Build history of the part. All positions in model axes, mm. A direction names the side the tool comes from. Give positions to 0.01 mm unless a question says otherwise; leave off trailing zeros. Use a Markdown table: item, result. Add a question column.
(1) Mould opens along Y. For faces 1 (the face through (30, 12, 40)), 2 (the face through (-0.901, -75.004, 24.79)), 3 (the face through (0.901, 75.004, 24.79)), 4 (the face through (-42.222, 32.375, 25.243)) say: +Y half, -Y half, draft (parallel to the pull), parting line (faces both ways), or undercut.
(2) Slice it at C-C (x = 69). Count the separate pieces of the cut face and the enclosed holes in it, then the cut area to 3 significant figures.
(3) Which spindle directions (+Z, -Z, +X, -X, +Y, -Y) get a long thin tool onto all of the face, cutting with end or side? Do faces 5 (the face through (-85.82, 0.79, 16.79)), 6 (the face through (92.5, -1, 7)), 7 (the face through (85.572, 0.791, 16.856)), 8 (the face through (-66.18, 86.51, 25.65)). Say none if no direction does.
(4) Wall check: line 1 (X direction, y = -86, z = 27); line 2 (Y direction, x = -64.5, z = 22); line 3 (X direction, y = -72, z = 4.5). Give the ranges that are in metal, low to high.
(5) Flat gauge pins, fed straight in: pin 1 (1.5 mm diameter, centred on x = 31.5, z = 6, fed in from -Y); pin 2 (10.5 mm diameter, centred on x = 75, y = 75, fed in from +Z); pin 3 (7.5 mm diameter, centred on y = 25, z = 11, fed in from -X); pin 4 (14.5 mm diameter, centred on x = 77, y = 74.5, fed in from +Z). Where does each tip first touch, or does it go through?
from build123d import *

# Parameters (mm, degrees)
SKETCH1_R                       = 25
BOSS_EXTRUDE1_DEPTH             = 30
SKETCH2_W                       = 185
SKETCH2_H                       = 185
BOSS_EXTRUDE2_DEPTH             = 15
DRAFT1_ANGLE                    = 15
DRAFT2_ANGLE                    = 15
DRAFT3_ANGLE                    = 15
DRAFT4_ANGLE                    = 15
SKETCH3_R                       = 42.5
BOSS_EXTRUDE3_DEPTH             = 40
CBORE_FOR_M16_SBHCS1_AT_2_COUNT = 2
CBORE_FOR_M16_SBHCS1_AT_2_PITCH = 150
CBORE_FOR_M16_SBHCS1_AT_3_COUNT = 2
CBORE_FOR_M16_SBHCS1_AT_3_PITCH = 150
CBORE_FOR_M16_SBHCS1_AT_4_COUNT = 2
CBORE_FOR_M16_SBHCS1_AT_4_PITCH = 212.132034356
SKETCH6_R                       = 30
CUT_EXTRUDE1_DEPTH              = 147.969384567
SKETCH7_R                       = 77.5
CUT_EXTRUDE2_DEPTH              = 5
FILLET1_R                       = 3
CHAMFER1_SIZE                   = 2


with BuildPart() as part:
    # Sketch1 → Boss-Extrude1 (new body)
    with BuildSketch(Plane.XY):
        with BuildLine():
            ThreePointArc((-60, 95), (-52.639320225, 86.180339887), (-50, 75))
            ThreePointArc((-50, 75), (-67.09430585, 51.282917549), (-95, 60))
            ThreePointArc((-95, 60), (-75, 0), (-95, -60))
            ThreePointArc((-95, -60), (-67.09430585, -51.282917549), (-50, -75))
            ThreePointArc((-50, -75), (-52.639320225, -86.180339887), (-60, -95))
            ThreePointArc((-60, -95), (0, -75), (60, -95))
            ThreePointArc((60, -95), (57.32233047, -57.32233047), (95, -60))
            ThreePointArc((95, -60), (75, 0), (95, 60))
            ThreePointArc((95, 60), (57.32233047, 57.32233047), (60, 95))
            ThreePointArc((60, 95), (0, 75), (-60, 95))
        make_face()
        with Locations((-75, 75)):
            Circle(SKETCH1_R)
        with Locations((75, 75)):
            Circle(SKETCH1_R)
        with Locations((75, -75)):
            Circle(SKETCH1_R)
        with Locations((-75, -75)):
            Circle(SKETCH1_R)
    extrude(amount=BOSS_EXTRUDE1_DEPTH)

    # Sketch2 → Boss-Extrude2 (add)
    with BuildSketch(Plane.XY):
        Rectangle(SKETCH2_W, SKETCH2_H)
    extrude(amount=BOSS_EXTRUDE2_DEPTH)

    # Draft1
    draft1_faces = [part.faces().sort_by_distance(p)[0] for p in [
        (85.444692503, 0, 15),
    ]]
    draft(draft1_faces, Plane(origin=(92.5, -92.5, 15), x_dir=(0, 0, 1), z_dir=(1, 0, 0)), DRAFT1_ANGLE)

    # Draft2
    draft2_faces = [part.faces().sort_by_distance(p)[0] for p in [
        (0, 85.444692503, 15),
    ]]
    draft(draft2_faces, Plane(origin=(-92.5, 92.5, 15), x_dir=(0, 0, 1), z_dir=(0, 1, 0)), DRAFT2_ANGLE)

    # Draft3
    draft3_faces = [part.faces().sort_by_distance(p)[0] for p in [
        (-85.444692503, 0, 15),
    ]]
    draft(draft3_faces, Plane(origin=(-92.5, -92.5, 15), x_dir=(0, 0, -1), z_dir=(-1, 0, 0)), DRAFT3_ANGLE)

    # Draft4
    draft4_faces = [part.faces().sort_by_distance(p)[0] for p in [
        (0, -85.444692503, 15),
    ]]
    draft(draft4_faces, Plane(origin=(-92.5, -92.5, 15), x_dir=(0, 0, -1), z_dir=(0, -1, 0)), DRAFT4_ANGLE)

    # Sketch3 → Boss-Extrude3 (add)
    with BuildSketch(Plane.XY):
        Circle(SKETCH3_R)
    extrude(amount=BOSS_EXTRUDE3_DEPTH)

    # Sketch5 → CBORE for M16 SBHCS1 (revolve, cut)
    with BuildSketch(Plane(origin=(-75, 75, 30), x_dir=(0, -1, 0), z_dir=(1, 0, 0))):
        Polygon((0, 0), (0, 30), (8.75, 30), (8.75, 8.8), (14.5, 8.8), (14.5, 0.025), (14.525, 0), align=None)
    cbore_for_m16_sbhcs1 = revolve(axis=Axis((-75, 75, 36.35), (0, 0, -1)), mode=Mode.SUBTRACT)

    # CBORE for M16 SBHCS1 at 2: CBORE for M16 SBHCS1 ×2
    with Locations(*[(i * CBORE_FOR_M16_SBHCS1_AT_2_PITCH, 0, 0) for i in range(1, CBORE_FOR_M16_SBHCS1_AT_2_COUNT)]):
        add(cbore_for_m16_sbhcs1, mode=Mode.SUBTRACT)

    # CBORE for M16 SBHCS1 at 3: CBORE for M16 SBHCS1 ×2
    with Locations(*[(0, -i * CBORE_FOR_M16_SBHCS1_AT_3_PITCH, 0) for i in range(1, CBORE_FOR_M16_SBHCS1_AT_3_COUNT)]):
        add(cbore_for_m16_sbhcs1, mode=Mode.SUBTRACT)

    # CBORE for M16 SBHCS1 at 4: CBORE for M16 SBHCS1 ×2
    with Locations(*[Vector(0.7071067811865476, -0.7071067811865476, 0) * (i * CBORE_FOR_M16_SBHCS1_AT_4_PITCH) for i in range(1, CBORE_FOR_M16_SBHCS1_AT_4_COUNT)]):
        add(cbore_for_m16_sbhcs1, mode=Mode.SUBTRACT)

    # Sketch6 → Cut-Extrude1 (cut, through all)
    with BuildSketch(Plane.XY.offset(40)):
        Circle(SKETCH6_R)
    extrude(amount=-CUT_EXTRUDE1_DEPTH, mode=Mode.SUBTRACT)

    # Sketch7 → Cut-Extrude2 (cut)
    with BuildSketch(Plane(origin=(0, 0, 0), x_dir=(-1, 0, 0), z_dir=(0, 0, -1))):
        Circle(SKETCH7_R)
    extrude(amount=-CUT_EXTRUDE2_DEPTH, mode=Mode.SUBTRACT)

    # Sketch8 → Cut-Revolve1 (revolve, cut)
    with BuildSketch(Plane(origin=(0, 0, 0), x_dir=(0, 0, -1), z_dir=(1, 0, 0)), mode=Mode.PRIVATE) as cut_revolve1_sk:
        Polygon((-30, 42.5), (-30, 60), (-25, 52.859259966), (-25, 42.5), align=None)
    revolve(cut_revolve1_sk.sketch.rotate(Axis((0, 0, 77.404119515), (0, 0, -1)), 90), axis=Axis((0, 0, 77.404119515), (0, 0, -1)), mode=Mode.SUBTRACT)

    # Fillet1
    fillet1_edges = [part.edges().sort_by_distance(p)[0] for p in [
        (-42.5, 0, 25),
    ]]
    fillet(fillet1_edges, radius=FILLET1_R)

    # Chamfer1
    chamfer1_edges = [part.edges().sort_by_distance(p)[0] for p in [
        (-30, 0, 40),
        (-30, 0, 5),
        (-42.5, 0, 40),
    ]]
    chamfer(chamfer1_edges, length=CHAMFER1_SIZE)


solid = part.part
Solution:
| question | item | result |
|---|---|---|
| 1 | face 1 | draft |
| 1 | face 2 | -Y half |
| 1 | face 3 | +Y half |
| 1 | face 4 | undercut |
| 2 | separate pieces | 3 |
| 2 | enclosed holes | 0 |
| 2 | area | 4,600 mm2 |
| 3 | face 5 | +Z, -X |
| 3 | face 6 | +Z, -Z, +X |
| 3 | face 7 | +Z, +X |
| 3 | face 8 | +Z |
| 4 | line 1 | -97.45 to -84.45, -65.55 to -45.6, 45.6 to 65.55, 84.45 to 97.45 |
| 4 | line 2 | -97.69 to -85, -65 to 65, 85 to 97.69 |
| 4 | line 3 | -99.82 to -83.22, -66.78 to -28.67, 28.67 to 66.78, 83.22 to 99.82 |
| 5 | pin 1 | y = -92.5 |
| 5 | pin 2 | through |
| 5 | pin 3 | x = -92.5 |
| 5 | pin 4 | z = 21.2 |
